Autodesk Inventor part; units mm, degrees
ref_plane "YZ Plane" through (0, 0, 0) normal (1, 0, 0) x (0, 1, 0)
ref_plane "XZ Plane" through (0, 0, 0) normal (0, 1, 0) x (-1, 0, 0)
ref_plane "XY Plane" through (0, 0, 0) normal (0, 0, 1) x (1, 0, 0)
sketch "Sketch1" plane through (0, 0, 0) normal (0, 1, 0) x (-1, 0, 0)
  circle A0 centre (0, 0) radius 10.75
  circle A1 centre (0, 0) radius 13.75
  dimension "d0" = 21.5
  dimension "d1" = 3
extrude "Extrusion1" add sketch "Sketch1" along normal blind 1.9
sketch "Sketch2" plane through (0, 1.9, 0) normal (0, 1, 0) x (1, 0, 0)
  circle A0 centre (0, 0) radius 13.75
extrude "Extrusion2" add sketch "Sketch2" along normal blind 2
sketch "Sketch3" plane through (0, 3.9, 0) normal (0, 1, 0) x (1, 0, 0)
  circle A0 centre (0, 0) radius 1.75
  dimension "d6" = 3.5
extrude "Extrusion3" cut sketch "Sketch3" along normal through all both and the other way through all
sketch "Sketch4" plane through (0, 1.9, 0) normal (0, -1, 0) x (1, 0, 0)
  circle A0 centre (7.5, 0.0066) radius 0.95
  circle A1 centre (7.5, -3.3934) radius 0.95
  circle A2 centre (7.5, 3.4066) radius 0.95
  point P0 (0, 0)
  dimension "d9" = 1.9
  dimension "d10" = 1.9
  dimension "d11" = 1.9
  dimension "d12" = 7.5
  dimension "d13" = 7.5
  dimension "d14" = 7.5
  dimension "d15" = 3.4
  dimension "d16" = 3.4
extrude "Extrusion4" [suppressed]
pattern_circular "Circular Pattern1" [suppressed]
sketch "Sketch5" plane through (0, 3.9, 0) normal (0, 1, 0) x (1, 0, 0)
  circle A0 centre (0, -17.85) radius 0.8
  circle A1 centre (0, -17.85) radius 1.45
  circle A2 centre (0, 0) radius 13.75
  line L0 (-1.2939, -18.5046) -> (-4, -13.1553)
  line L1 (1.2939, -18.5046) -> (4, -13.1553)
  dimension "d22" = 1.6
  dimension "d23" = 17.85
  dimension "d24" = 2.9
  dimension "d25" = 0
  dimension "d26" = 4
  dimension "d27" = 4
extrude "Extrusion5" add sketch "Sketch5" against normal blind 2 contours A1 | A1 L0 A2 L1
sketch "Sketch6" plane through (0, 3.9, 0) normal (0, 1, 0) x (1, 0, 0)
  circle A0 centre (0, 0) radius 14.35
  dimension "d30" = 28.7
extrude "Extrusion6" add sketch "Sketch6" along normal blind 4
sketch "Sketch7" plane through (0, 7.9, 0) normal (0, 1, 0) x (1, 0, 0)
  circle A0 centre (0, 0) radius 1.75
  line L0 (0, 0) -> (0, -16.57)
  line L1 (0, -16.57) -> (7.1751, -12.4274)
  line L2 (7.1751, -12.4274) -> (0, 0)
  circle A1 centre (0, 0) radius 14.35
  arc A2 (7.1751, -12.4274) -> (-7.1751, -12.4274) centre (0, -16.57) ccw
  arc A3 (-7.1751, -12.4274) -> (7.1751, -12.4274) centre (0, 0) ccw
  dimension "d33" = 16.57
extrude "Extrusion7" cut sketch "Sketch7" against normal blind 4 contours A2 A1 L0 | L0 A1 A2
sketch "Sketch8" plane through (0, 1.9, 0) normal (0, -1, 0) x (1, 0, 0)
  circle A0 centre (-3.4066, 7.5) radius 0.95
  arc A1 (-7.1751, 12.4274) -> (-6.8562, 11.9187) centre (0, 16.57) ccw
  circle A2 centre (-0.0066, 7.5) radius 0.95
  circle A3 centre (3.3934, 7.5) radius 0.95
  circle A4 centre (7.5, 3.4066) radius 0.95
  circle A5 centre (7.5, 0.0066) radius 0.95
  circle A6 centre (7.5, -3.3934) radius 0.95
  circle A7 centre (3.4066, -7.5) radius 0.95
  circle A8 centre (0.0066, -7.5) radius 0.95
  circle A9 centre (-3.3934, -7.5) radius 0.95
  circle A10 centre (-7.5, -3.4066) radius 0.95
  circle A11 centre (-7.5, -0.0066) radius 0.95
  circle A12 centre (-7.5, 3.3934) radius 0.95
  circle A13 centre (0, 0) radius 1.75
  arc A14 (-7.1751, 12.4274) -> (7.1751, 12.4274) centre (0, 0) ccw
  arc A15 (6.8562, 11.9187) -> (7.1751, 12.4274) centre (0, 16.57) ccw
  arc A16 (-6.8562, 11.9187) -> (6.8562, 11.9187) centre (0, 0) ccw
  point P0 (0.5052, 8.3003)
  point P1 (-0.5172, 8.3011)
extrude "Extrusion8" [suppressed]
sketch "Sketch9" plane through (0, 1.9, 0) normal (0, -1, 0) x (1, 0, 0)
  circle A0 centre (0, 0) radius 3.75
  dimension "d38" = 7.5
extrude "Extrusion9" cut sketch "Sketch9" against normal through all
sketch "Sketch10" plane through (0, 1.9, 0) normal (0, -1, 0) x (1, 0, 0)
  circle A0 centre (7.5, 3.4) radius 1.05
  circle A1 centre (7.5, 0) radius 1.05
  circle A2 centre (7.5, -3.4) radius 1.05
  point P0 (0, 0)
  dimension "d41" = 2.1
  dimension "d42" = 2.1
  dimension "d43" = 2.1
  dimension "d44" = 0
  dimension "d45" = 7.5
  dimension "d46" = 7.5
  dimension "d47" = 7.5
  dimension "d48" = 3.4
  dimension "d49" = 3.4
extrude "Extrusion10" cut sketch "Sketch10" against normal through all
pattern_circular "Circular Pattern2" [suppressed]
pattern_circular "Circular Pattern4" count 2 over 360 about axis through (0, -10, 0) along (0, 1, 0) of "Extrusion10"
sketch "Sketch11" plane through (0, 7.9, 0) normal (0, 1, 0) x (1, 0, 0)
  circle A0 centre (7.5, -3.4) radius 1.05
  circle A1 centre (7.5, 0) radius 1.05
  circle A2 centre (7.5, 3.4) radius 1.05
  circle A3 centre (7.5, -3.4) radius 1.65
  circle A4 centre (7.5, 0) radius 1.65
  circle A5 centre (7.5, 3.4) radius 1.65
  point P0 (0, 0)
  dimension "d61" = 3.3
  dimension "d62" = 3.3
  dimension "d63" = 3.3
extrude "Extrusion11" cut sketch "Sketch11" against normal blind 3 contours A0 | A1 | A2 | A3 | A4 | A5
pattern_circular "Circular Pattern5" count 2 over 360 about axis through (0, -10, 0) along (0, 1, 0) of "Extrusion11"
pattern_circular "Circular Pattern6" [suppressed]
mirror "Mirror1" about plane through (0, 0, 0) normal (0, 0, 1) of "Extrusion5"
mirror "Mirror2" about plane through (0, 0, 0) normal (0, 0, 1) of "Extrusion7"
equation "\"d16\" = d15"
equation "\"d49\" = d48"
properties part number "pin_r1"
Geometry: final body of the model. Coordinates: model frame, mm. A direction names the side the tool comes from. Coordinates: 2 decimals unless noted, no trailing zeros. Order: outer loops, then holes, each group sorted by start corner. A loop starts at its lowest first (then second) coordinate and runs counter-clockwise, first axis right, second up. Notation, with made-up numbers: (65.25, 14) -> (124.25, 14) arc R27 cw to (124.25, 33) -> close; hole circle Ø10 at (55, -33.75). An arc over 180 degrees is marked (long way). Write each question's results on one line, items separated by ' | '. Start each with the question number.
1) Cut plane C-C, the plane z = -3. State how many separate pieces and enclosed holes the cut face has, and give its area (3 significant figures).
2) First-contact query: pin 1 (6 mm diameter, centred on x = 0, z = 0, fed in from +Y); pin 2 (2.5 mm diameter, centred on x = 7.5, z = -3.4, fed in from -Y); pin 3 (9 mm diameter, centred on x = 1, z = 16, fed in from +Y); pin 4 (4 mm diameter, centred on x = 10, y = 1.5, fed in from +Z). Flat tips, straight axial feed; report the tip coordinate or a pass-through.
3) Cut plane D-D, the plane z = 17.85. Output: boundary loops of the cut face in (x, y).
4) Cut plane A-A, the plane x = 0. Output: boundary loops of the cut face in (y, z).
5) Cut plane B-B, the plane y = 6.5. Output: boundary loops of the cut face in (x, z), and give its area (3 significant figures).
6) Set-up query: faces 5 (the flat face through (0, 3.9, 12)), 6 (the cylindrical face through (-6.19, 6.42, 2.4)), 7 (the flat face through (14, 3.9, 0)). Return all of +Z, -Z, +X, -X, +Y, -Y with unobstructed straight access to the full face (end or side cutting, diameter ignored); none if empty.
7) Material intervals for line 1 along Z through (x, y) = (7.5, 3.25); line 2 along Z through (x, y) = (-7.25, 2.5); line 3 along X through (y, z) = (5, -4), sorted ascending.
8) Mould query, pull axis X, two halves, no side actions, for faces 1 (the cylindrical face through (0, 2.9, -19.3)), 2 (the flat face through (0, 1.9, 5)), 3 (the flat face through (0, 1.9, 16)), 4 (the flat face through (2.628, 2.914, 15.867)). Classes: released by +X, released by -X, zero draft, split by the parting line, or undercut.
Checks:
1) separate pieces: 4 | enclosed holes: 0 | area: 120 mm^2
2) pin 1: through | pin 2: y = 1.9 | pin 3: y = 3.9 | pin 4: z = 11.18
3) outline: (-1.63, 1.9) -> (-0.8, 1.9) -> (-0.8, 3.9) -> (-1.63, 3.9) -> close; (0.8, 1.9) -> (1.63, 1.9) -> (1.63, 3.9) -> (0.8, 3.9) -> close
4) outline: (0, -13.75) -> (1.9, -13.75) -> (1.9, -17.05) -> (3.9, -17.05) -> (3.9, -8.28) -> (7.9, -8.28) -> (7.9, -3.75) -> (1.9, -3.75) -> (1.9, -10.75) -> (0, -10.75) -> close; (0, 10.75) -> (1.9, 10.75) -> (1.9, 3.75) -> (7.9, 3.75) -> (7.9, 8.28) -> (3.9, 8.28) -> (3.9, 17.05) -> (1.9, 17.05) -> (1.9, 13.75) -> (0, 13.75) -> close; (1.9, -19.3) -> (3.9, -19.3) -> (3.9, -18.65) -> (1.9, -18.65) -> close; (1.9, 18.65) -> (3.9, 18.65) -> (3.9, 19.3) -> (1.9, 19.3) -> close
5) outline: (-7.18, -12.43) arc R8.29 cw to (7.18, -12.43) arc R14.35 ccw to (7.18, 12.43) arc R8.29 cw to (-7.18, 12.43) arc R14.35 ccw to start; hole circle Ø3.3 at (-7.5, -3.4); hole circle Ø3.3 at (-7.5, 0); hole circle Ø3.3 at (-7.5, 3.4); hole circle Ø7.5 at (0, 0); hole circle Ø3.3 at (7.5, -3.4); hole circle Ø3.3 at (7.5, 0); hole circle Ø3.3 at (7.5, 3.4) | area: 430 mm^2
6) face 5: +Z, +Y | face 6: +Y | face 7: +X, -Y
7) line 1: -11.52 to -4.45, -2.35 to -1.05, 1.05 to 2.35, 4.45 to 11.52 | line 2: -11.68 to -4.42, -2.38 to -1.02, 1.02 to 2.38, 4.42 to 11.68 | line 3: -13.78 to -9.04, -5.96 to 5.96, 9.04 to 13.78
8) face 1: split by the parting line | face 2: undercut | face 3: zero draft | face 4: released by +X
